from build123d import *

# Parameters (mm, degrees)
CROQUIS1_W                   = 63.5
CROQUIS1_H                   = 38.1
SALIENTE_EXTRUIR1_DEPTH      = 50.8
CROQUIS2_R                   = 12.7
CORTAR_EXTRUIR1_DEPTH        = 63.5
CROQUIS3_R                   = 9.525
CORTAR_EXTRUIR2_DEPTH        = 63.5
REDONDEO1_R                  = 2.54
TALADRO_ROSCADO_10_322_D     = 4.0386
TALADRO_ROSCADO_10_322_DEPTH = 13.6144
TALADRO_ROSCADO_10_322_TIP   = 1.213317848
TALADRO_ROSCADO_10_321_D     = 4.0386
TALADRO_ROSCADO_10_321_DEPTH = 13.6144
TALADRO_ROSCADO_10_321_TIP   = 1.213317848


with BuildPart() as part:
    # Croquis1 → Saliente-Extruir1 (new body)
    with BuildSketch(Plane(origin=(0, 0, 0), x_dir=(1, 0, 0), z_dir=(0, 1, 0))):
        Rectangle(CROQUIS1_W, CROQUIS1_H)
    extrude(amount=SALIENTE_EXTRUIR1_DEPTH)

    # Croquis2 → Cortar-Extruir1 (cut)
    with BuildSketch(Plane.XY.offset(19.05)):
        with Locations((-11.43, 25.4)):
            Circle(CROQUIS2_R)
    extrude(amount=-CORTAR_EXTRUIR1_DEPTH, mode=Mode.SUBTRACT)

    # Croquis3 → Cortar-Extruir2 (cut)
    with BuildSketch(Plane(origin=(0, 50.8, 0), x_dir=(1, 0, 0), z_dir=(0, 1, 0))):
        with Locations(Location((14.605, 0, 0), (0, 0, 270))):
            Circle(CROQUIS3_R)
    extrude(amount=-CORTAR_EXTRUIR2_DEPTH, mode=Mode.SUBTRACT)

    # Redondeo1
    redondeo1_edges = [part.edges().sort_by_distance(p)[0] for p in [
        (-31.75, 50.8, 0),
        (0, 50.8, 19.05),
        (31.75, 50.8, 0),
        (0, 0, 19.05),
        (-31.75, 0, 0),
        (0, 0, -19.05),
        (31.75, 0, 0),
        (0, 50.8, -19.05),
        (31.75, 25.4, 19.05),
        (-31.75, 25.4, 19.05),
        (-31.75, 25.4, -19.05),
        (31.75, 25.4, -19.05),
    ]]
    fillet(redondeo1_edges, radius=REDONDEO1_R)

    # Taladro roscado #10-322
    with Locations(Plane(origin=(31.75, 0, 0), x_dir=(0, 0, -1), z_dir=(1, 0, 0))):
        with Locations((0, 25.4)):
            Hole(TALADRO_ROSCADO_10_322_D / 2, depth=TALADRO_ROSCADO_10_322_DEPTH)
            with Locations((0, 0, -(TALADRO_ROSCADO_10_322_DEPTH + TALADRO_ROSCADO_10_322_TIP / 2))):  # 118° drill point
                Cone(0, TALADRO_ROSCADO_10_322_D / 2, TALADRO_ROSCADO_10_322_TIP, mode=Mode.SUBTRACT)

    # Taladro roscado #10-321
    with Locations(Plane.ZY.offset(31.75)):
        with Locations((0, 25.4)):
            Hole(TALADRO_ROSCADO_10_321_D / 2, depth=TALADRO_ROSCADO_10_321_DEPTH)
            with Locations((0, 0, -(TALADRO_ROSCADO_10_321_DEPTH + TALADRO_ROSCADO_10_321_TIP / 2))):  # 118° drill point
                Cone(0, TALADRO_ROSCADO_10_321_D / 2, TALADRO_ROSCADO_10_321_TIP, mode=Mode.SUBTRACT)


solid = part.part
Can you work these out from the model? Positions are in its coordinate system, mm. A direction names the side the tool comes from. Give positions to 0.01 mm unless a question says otherwise; leave off trailing zeros. Loops run counter-clockwise (first coordinate to the right, second up) from the corner with the lowest first, then second, coordinate; pieces in that order, holes last. Notation, with made-up numbers: (-10, 65) - (25, 65) arc R30 ccw to (25, 103) - close; hole circle Ø2 at (25.25, 31). An arc over 180 degrees is marked (long way). One line per item, written item: value.
(1) If we section it at A-A, the plane z = 0: List the corners of the cut face in (x, y) for me, plus the area to 3 significant figures.
Verdict:
outline: (-31.75, 2.54) arc R2.54 ccw to (-29.21, 0) - (5.08, 0) - (5.08, 50.8) - (-29.21, 50.8) arc R2.54 ccw to (-31.75, 48.26) - (-31.75, 27.42) - (-23.97, 27.42) arc R12.7 cw (long way) to (-23.97, 23.38) - (-31.75, 23.38) - close; (24.13, 0) - (29.21, 0) arc R2.54 ccw to (31.75, 2.54) - (31.75, 23.38) - (24.13, 23.38) - close; (24.13, 27.42) - (31.75, 27.42) - (31.75, 48.26) arc R2.54 ccw to (29.21, 50.8) - (24.13, 50.8) - close
area: 1,680 mm^2
(2) I need wall thicknesses on line 1 along Y through (x, z) = (-11, 5); line 2 along X through (y, z) = (5, -0.5); line 3 along Y through (x, z) = (-29, 0). Which ranges of each line are inside material? Lowest first, please.
Verdict:
line 1: 0 to 12.71, 38.09 to 50.8
line 2: -31.75 to 5.09, 24.12 to 31.75
line 3: 0 to 23.38, 27.42 to 50.8
(3) If we section it at C-C, the plane y = 25.4: State how many separate pieces and enclosed holes the cut face has, plus the area to 3 significant figures.
Verdict:
separate pieces: 3
enclosed holes: 0
area: 1,100 mm^2
(4) I'm going to push flat-ended pins straight in: pin 1 (2.5 mm diameter, centred on y = 25.4, z = 0, fed in from +X); pin 2 (3 mm diameter, centred on y = 25.4, z = 0, fed in from -X). Where does each tip first touch, or does it pass through?
Verdict:
pin 1: x = 5.16
pin 2: x = 1.18
(5) If we section it at D-D, the plane x = -11.43: List the corners of the cut face in (y, z) for me.
Verdict:
outline: (0, -16.51) arc R2.54 ccw to (2.54, -19.05) - (12.7, -19.05) - (12.7, 19.05) - (2.54, 19.05) arc R2.54 ccw to (0, 16.51) - close; (38.1, -19.05) - (48.26, -19.05) arc R2.54 ccw to (50.8, -16.51) - (50.8, 16.51) arc R2.54 ccw to (48.26, 19.05) - (38.1, 19.05) - close
(6) If we mould it in two halves opening along Y, with no side actions, what happens to faces 3 (the face through (0.409, 50.036, -18.326)), 4 (the face through (0.409, 0.764, -18.326)), 5 (the face through (0.684, 29.215, 0.267))? For each: released by +Y, released by -Y, zero draft, split by the parting line, or undercut.
Verdict:
face 3: released by +Y
face 4: released by -Y
face 5: undercut
(7) On a 3-axis mill with a long thin cutter (end or side, diameter ignored), from which of +Z, -Z, +X, -X, +Y, -Y can I reach the whole of each face in a straight line? I mean faces 1 (the face through (-31.75, 25, -3)), 2 (the face through (-27.805, 27.402, 0.263)). Say none if no direction works.
Verdict:
face 1: +Z, -Z, -X, +Y, -Y
face 2: -X
(8) If we section it at B-B, the plane y = 33.5: List the corners of the cut face in (x, z) for me (3 decimals).
Verdict:
outline: (-31.75, -16.51) arc R2.54 ccw to (-29.21, -19.05) - (-21.212, -19.05) - (-21.212, 19.05) - (-29.21, 19.05) arc R2.54 ccw to (-31.75, 16.51) - close; (-1.648, -19.05) - (29.21, -19.05) arc R2.54 ccw to (31.75, -16.51) - (31.75, 16.51) arc R2.54 ccw to (29.21, 19.05) - (-1.648, 19.05) - close; hole circle Ø19.05 at (14.605, 0)
